```python
from build123d import *

# Parameters (mm, degrees)
SKETCH2_W           = 127
SKETCH2_H           = 19.05
BOSS_EXTRUDE1_DEPTH = 6.35
SKETCH3_W           = 16.857329018
SKETCH3_H           = 3.81675374
CUT_EXTRUDE1_DEPTH  = 6.35
CUT_EXTRUDE2_DEPTH  = 7.35
SKETCH5_R           = 2.208058356
CUT_EXTRUDE3_DEPTH  = 6.35


with BuildPart() as part:
    # Sketch2 → Boss-Extrude1 (new body)
    with BuildSketch(Plane(origin=(0, 0, 0), x_dir=(1, 0, 0), z_dir=(0, 1, 0))):
        Rectangle(SKETCH2_W, SKETCH2_H)
    extrude(amount=BOSS_EXTRUDE1_DEPTH)

    # Sketch3 → Cut-Extrude1 (cut)
    with BuildSketch(Plane(origin=(63.5, 0, 0), x_dir=(0, 0, -1), z_dir=(1, 0, 0))):
        with Locations((0, 3.343970869)):
            Rectangle(SKETCH3_W, SKETCH3_H)
    extrude(amount=-CUT_EXTRUDE1_DEPTH, mode=Mode.SUBTRACT)

    # Sketch4 → Cut-Extrude2 (cut, through all)
    with BuildSketch(Plane(origin=(0, 6.35, 0), x_dir=(1, 0, 0), z_dir=(0, 1, 0))):
        Polygon((-22.637713534, -4.636428392), (-4.505889832, -6.062078542), (-4.505889832, -7.487728691), (-61.757195928, -7.487728691), (-61.757195928, -4.636428392), align=None)
    extrude(amount=-CUT_EXTRUDE2_DEPTH, mode=Mode.SUBTRACT)

    # Sketch5 → Cut-Extrude3 (cut)
    with BuildSketch(Plane(origin=(0, 6.35, 0), x_dir=(1, 0, 0), z_dir=(0, 1, 0))):
        with Locations((-43.986162308, 2.214937446)):
            Circle(SKETCH5_R)
    extrude(amount=-CUT_EXTRUDE3_DEPTH, mode=Mode.SUBTRACT)


solid = part.part
```
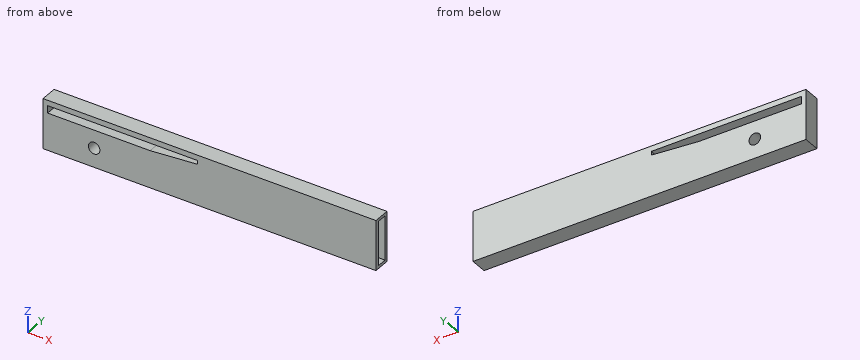
Build history of the part. All positions in model axes, mm. Give positions to 0.01 mm unless a question says otherwise; leave off trailing zeros. Loops run counter-clockwise (first coordinate to the right, second up) from the corner with the lowest first, then second, coordinate; pieces in that order, holes last.
Item 1: Slice it at C-C, the plane y = 2.75. List the corners of the cut face in (x, z) (3 decimals), and give its area (3 significant figures).
Answers follow:
outline: (-63.5, -9.525) - (63.5, -9.525) - (63.5, -8.429) - (57.15, -8.429) - (57.15, 8.429) - (63.5, 8.429) - (63.5, 9.525) - (-63.5, 9.525) - close; hole (-61.757, 4.636) - (-22.638, 4.636) - (-4.506, 6.062) - (-4.506, 7.488) - (-61.757, 7.488) - close; hole circle Ø4.416 at (-43.986, -2.215)
area: 2,150 mm2
Item 2: Drill centre lines: line 1 (X direction, y = 2.5, z = -2); line 2 (X direction, y = 1.25, z = 7); line 3 (X direction, y = 4.5, z = 8). Where is each one in solid material? Low to high.
Answers follow:
line 1: x = -63.5 to -46.18, -41.79 to 57.15
line 2: x = -63.5 to -61.76, -4.51 to 63.5
line 3: x = -63.5 to 57.15
Item 3: Slice it at A-A, the plane x = -38. List the corners of the cut face in (y, z) (3 decimals), and give its area (3 significant figures).
Answers follow:
outline: (0, -9.525) - (6.35, -9.525) - (6.35, 4.636) - (0, 4.636) - close; (0, 7.488) - (6.35, 7.488) - (6.35, 9.525) - (0, 9.525) - close
area: 103 mm2
Item 4: Flat gauge pins, fed straight in: pin 1 (6 mm diameter, centred on x = 14.5, z = -7.5, fed in from -Y); pin 2 (1.5 mm diameter, centred on y = 2.5, z = 6.5, fed in from +X). Where does each tip first touch, or does it go through?
Answers follow:
pin 1: stops at y = 0
pin 2: stops at x = 57.15
Item 5: Slice it at B-B, the plane z = 2.25. List the corners of the cut face in (x, y).
Answers follow:
outline: (-63.5, 0) - (63.5, 0) - (63.5, 1.44) - (57.15, 1.44) - (57.15, 5.25) - (63.5, 5.25) - (63.5, 6.35) - (-63.5, 6.35) - close
